Autodesk Inventor part; units mm, degrees
ref_plane "YZ Plane" through (0, 0, 0) normal (1, 0, 0) x (0, 1, 0)
ref_plane "XZ Plane" through (0, 0, 0) normal (0, 1, 0) x (-1, 0, 0)
ref_plane "XY Plane" through (0, 0, 0) normal (0, 0, 1) x (1, 0, 0)
sketch "スケッチ1" plane through (0, 0, 0) normal (0, 1, 0) x (-1, 0, 0)
  line L0 (0, 0) -> (107, 0)
  line L1 (107, 0) -> (107, -165)
  line L2 (107, -165) -> (0, -165)
  line L3 (0, -165) -> (0, 0)
  line L4 (107, 0) -> (114.96, 0)
  line L5 (114.96, 0) -> (114.96, -8)
  line L6 (114.96, -8) -> (107, -8)
  line L7 (107, -8) -> (107, 0)
  line L8 (53.5, 0) -> (53.5, -165)
  circle A0 centre (111.35, -4) radius 1.75
  line L9 (107, -82.5) -> (0, -82.5)
  circle A1 centre (110.96, -4) radius 4
  line L10 (107, -165) -> (114.96, -165)
  line L11 (114.96, -157) -> (107, -157)
  circle A2 centre (111.35, -161) radius 1.75
  circle A3 centre (110.96, -161) radius 4
  line L12 (0, 0) -> (-7.96, 0)
  line L13 (-7.96, -8) -> (0, -8)
  circle A4 centre (-4.35, -4) radius 1.75
  circle A5 centre (-3.96, -4) radius 4
  circle A6 centre (-3.96, -161) radius 4
  circle A7 centre (-4.35, -161) radius 1.75
  line L14 (-7.96, -157) -> (0, -157)
  line L15 (0, -165) -> (-7.96, -165)
  point P0 (109.6, -4)
  point P1 (110.96, -8)
  point P2 (110.96, 0)
  point P3 (-3.96, 0)
  point P4 (-3.96, -8)
  point P5 (-3.96, -157)
  point P6 (-3.96, -165)
  point P7 (110.96, -165)
  point P8 (110.96, -157)
  point P9 (0, -4.5643)
  point P10 (0, -3.4357)
  point P11 (107, -4.5643)
  point P12 (107, -3.4357)
  dimension "d6" = 3.5
  dimension "d0" = 107
  dimension "d1" = 165
  dimension "d2" = 8
  dimension "d3" = 7.96
  dimension "d5" = 56.1
  dimension "d7" = 8
extrude "押し出し1" add sketch "スケッチ1" along normal blind 1.7 contours L0 L8 L9 L3 A5 | L3 A5 L12 | L0 L1 A1 L9 L8 | A5 L3 | L3 A5 | L4 A1 L1 | L9 L1 A3 L2 L8 | L8 L2 L3 A6 L9 | L3 L13 A5 | A1 L1 | L1 A1 | A1 L6 L1 | L1 A3 L10 | L15 A6 L3 | L11 A3 L1 | L3 A6 L14 | A3 L1 | L1 A3 | A6 L3 | L3 A6
sketch "スケッチ2" plane through (0, 1.7, 0) normal (0, 1, 0) x (1, 0, 0)
  arc A0 (-110.96, 8) -> (-110.96, 0) centre (-110.96, 4) ccw
  line L0 (-110.96, 0) -> (3.96, 0)
  arc A1 (3.96, 0) -> (3.96, 8) centre (3.96, 4) ccw
  line L1 (3.96, 8) -> (0, 8)
  line L2 (0, 8) -> (0, 157)
  line L3 (0, 157) -> (3.96, 157)
  arc A2 (3.96, 157) -> (3.96, 165) centre (3.96, 161) ccw
  line L4 (3.96, 165) -> (-110.96, 165)
  arc A3 (-110.96, 165) -> (-110.96, 157) centre (-110.96, 161) ccw
  line L5 (-110.96, 157) -> (-107, 157)
  line L6 (-107, 157) -> (-107, 8)
  line L7 (-107, 8) -> (-110.96, 8)
  circle A4 centre (4.35, 161) radius 1.75
  circle A5 centre (4.35, 4) radius 1.75
  circle A6 centre (-111.35, 161) radius 1.75
  circle A7 centre (-111.35, 4) radius 1.75
  line L8 (-103.65, -0.9) -> (-3.35, -0.9)
  line L9 (-3.35, -0.9) -> (-3.35, 165.9)
  line L10 (-3.35, 165.9) -> (-103.65, 165.9)
  line L11 (-103.65, 165.9) -> (-103.65, -0.9)
  line L12 (-103.65, -0.9) -> (-3.35, 165.9) construction
  line L13 (-3.35, -0.9) -> (-103.65, 165.9) construction
  point P0 (0, 0)
  point P1 (-53.5, 82.5)
  dimension "d10" = 100.3
  dimension "d11" = 53.5
  dimension "d12" = 82.5
  dimension "d13" = 166.8
extrude "押し出し2" add sketch "スケッチ2" along normal blind 5.3 contours L11 L4 L9 L0 | L0 L9 L8 L11 | L11 L10 L9 L4
sketch "スケッチ3" plane through (0, 0, 0) normal (0, -1, 0) x (1, 0, 0)
  arc A0 (-110.96, 0) -> (-110.96, -8) centre (-110.96, -4) ccw
  line L0 (-107, -8) -> (-110.96, -8)
  line L1 (-107, -157) -> (-107, -8)
  line L2 (-110.96, -157) -> (-107, -157)
  arc A1 (-110.96, -157) -> (-110.96, -165) centre (-110.96, -161) ccw
  line L3 (3.96, -165) -> (-110.96, -165)
  arc A2 (3.96, -165) -> (3.96, -157) centre (3.96, -161) ccw
  line L4 (0, -157) -> (3.96, -157)
  line L5 (0, -8) -> (0, -157)
  line L6 (3.96, -8) -> (0, -8)
  arc A3 (3.96, -8) -> (3.96, 0) centre (3.96, -4) ccw
  line L7 (-110.96, 0) -> (3.96, 0)
  circle A4 centre (4.35, -161) radius 1.75
  circle A5 centre (4.35, -4) radius 1.75
  circle A6 centre (-111.35, -161) radius 1.75
  circle A7 centre (-111.35, -4) radius 1.75
  line L8 (-89, -36) -> (-20, -36)
  line L9 (-20, -36) -> (-20, -130)
  line L10 (-20, -130) -> (-89, -130)
  line L11 (-89, -130) -> (-89, -36)
  circle A8 centre (-23.5, -39.5) radius 1.75
  line L12 (-20, -83) -> (-89, -83)
  line L13 (-54.5, -130) -> (-54.5, -36)
  circle A9 centre (-23.5, -126.5) radius 1.75
  circle A10 centre (-85.5, -39.5) radius 1.75
  circle A11 centre (-85.5, -126.5) radius 1.75
  point P0 (0, 0)
  point P1 (-54.5, -83)
  dimension "d16" = 94
  dimension "d17" = 69
  dimension "d18" = 36
  dimension "d19" = 20
  dimension "d22" = 34.5
  dimension "d23" = 47
  dimension "d24" = 3.5
  dimension "d25" = 3.5
  dimension "d26" = 3.5
extrude "押し出し3" add sketch "スケッチ3" along normal blind 26 contours L8 L13 L12 L11 | L8 L9 L12 L13 | L12 L13 L10 L11 | L12 L9 L10 L13
ref_plane "作業平面1" through (-53.5, 1.7, 0) normal (1, 0, 0) x (0, 0, -1)
properties part number "Display_EVICIV7Inch"
For this review, take the finished solid that the model builds, in its own axes (mm). A direction names the side the tool comes from. Round coordinates to 2 decimals unless told otherwise and drop trailing zeros. Loops run counter-clockwise (first coordinate to the right, second up) from the corner with the lowest first, then second, coordinate; pieces in that order, holes last.
Q1. Add section A-A on z = -4. Write out the cut boundary in (x, y), plus the area to 3 significant figures.
Result sheet:
outline: (-114.96, 0) - (-113.1, 0) - (-113.1, 1.7) - (-114.96, 1.7) - close; (-109.6, 0) - (2.6, 0) - (2.6, 1.7) - (-3.35, 1.7) - (-3.35, 7) - (-103.65, 7) - (-103.65, 1.7) - (-109.6, 1.7) - close; (6.1, 0) - (7.96, 0) - (7.96, 1.7) - (6.1, 1.7) - close
area: 729 mm2
Q2. Machinability: for faces 5 (the face through (-85, 0, -39)), 6 (the face through (-89, -13, -84)), 7 (the face through (-103.65, 4, -84)), 8 (the face through (-1, 1.7, -82)), 9 (the face through (-20, -13, -82)), which of the approach directions +Z, -Z, +X, -X, +Y, -Y give a long, thin tool a straight path to every point of the face, cutting with its end or side? Answer none if there is none.
Result sheet:
face 5: -Y
face 6: +Z, -Z, -X, -Y
face 7: +Z, -Z, -X, +Y
face 8: +Z, -Z, +X, +Y
face 9: +Z, -Z, +X, -Y
Q3. Mouldability with a two-part tool opening along X and no side actions: class faces 1 (the face through (-23.88, -12.82, -124.79)), 2 (the face through (7.96, 0.84, -161.09)), 3 (the face through (-106, 1.7, -70)), 4 (the face through (-114.96, 0.84, -3.91)) as +X half, -X half, draft (parallel to the pull), parting line (faces both ways), or undercut.
Result sheet:
face 1: undercut
face 2: +X half
face 3: draft
face 4: -X half
Q4. Add section B-B on y = -18. Write out the cut boundary in (x, z), plus the area to 3 significant figures.
Result sheet:
outline: (-89, -130) - (-20, -130) - (-20, -36) - (-89, -36) - close; hole circle Ø3.5 at (-85.5, -126.5); hole circle Ø3.5 at (-85.5, -39.5); hole circle Ø3.5 at (-23.5, -126.5); hole circle Ø3.5 at (-23.5, -39.5)
area: 6,450 mm2
Q5. Insertion check: pin 1 Ø3 at (x, z) = (-85.5, -126.5) entering from -Y; pin 2 Ø1.5 at (x, y) = (-64, -4.5) entering from -Z; pin 3 Ø4 at (x, z) = (-111.35, -4) entering from +Y. Each pin has a flat end and moves straight along its axis. Give the tip position at first contact, or say it passes through.
Result sheet:
pin 1: stops at y = 0
pin 2: stops at z = -130
pin 3: stops at y = 1.7
Q6. To check wall thickness, follow line 1 along Z through (x, y) = (4, 1); line 2 along Z through (x, y) = (-85.5, -13.75); line 3 along X through (y, z) = (0.55, -161). State the ranges of each line that lie inside material, in increasing order.
Result sheet:
line 1: z = -165 to -162.71, -159.29 to -157, -8 to -5.71, -2.29 to 0
line 2: z = -130 to -128.25, -124.75 to -41.25, -37.75 to -36
line 3: x = -114.96 to -113.1, -109.6 to 2.6, 6.1 to 7.96
Q7. Add section D-D on z = -24. Write out the cut boundary in (x, y).
Result sheet:
outline: (-107, 0) - (0, 0) - (0, 1.7) - (-3.35, 1.7) - (-3.35, 7) - (-103.65, 7) - (-103.65, 1.7) - (-107, 1.7) - close
Q8. Add section C-C on x = -85.5. Write out the cut boundary in (y, z).
Result sheet:
outline: (-26, -130) - (0, -130) - (0, -165) - (1.7, -165) - (1.7, -165.9) - (7, -165.9) - (7, 0.9) - (1.7, 0.9) - (1.7, 0) - (0, 0) - (0, -36) - (-26, -36) - (-26, -37.75) - (0, -37.75) - (0, -41.25) - (-26, -41.25) - (-26, -124.75) - (0, -124.75) - (0, -128.25) - (-26, -128.25) - close
